Verification items for this drawing (mm, ordinates from the low corner). A direction names the side the tool comes from. Round coordinates to 2 decimals unless told otherwise and drop trailing zeros. Order: outer loops, then holes, each group sorted by start corner. A loop starts at its lowest first (then second) coordinate and runs counter-clockwise, first axis right, second up. Notation, with made-up numbers: (-2.5, -6.75) -> (24.5, -6.75) arc R16 cw to (24.5, 8.25) -> close; hole circle Ø3 at (-7, 41). An arc over 180 degrees is marked (long way). Return JSON: item names as keys, results as strings. Group by question number.
Item 1: Sectioned sample at A-A on z = 268.5. Record the cut outline in (x, y).
Item 2: Sectioned sample at D-D on z = 176.5. Record the cut outline in (x, y), plus the area to 3 significant figures.
Item 3: Depth check by flat-ended pin: pin 1 Ø1 at (y, z) = (60, 263) entering from -X; pin 2 Ø6 at (x, y) = (427, 50) entering from +Z; pin 3 Ø12 at (x, y) = (158.5, 15.5) entering from -Z. Enter the tip coordinate at first touch or a pass-through.
Item 4: Draft check along Z on the marked faces 1, 2 and 3. Enter one of: pulls with the +Z half, pulls with the -Z half, needs draft (parallel to the pull), parting line crosses it, or undercut.
Item 5: Scan lines: probe 1 along X at (y, z) = (39, 124.5); probe 2 along X at (y, z) = (17, 221.5); probe 3 along X at (y, z) = (36, 222). Record each from-to range of solid material in increasing order. Write a range as from..to.
Item 6: Access from +Z, -Z, +X, -X, +Y, -Y to the whole of each face (thin tool, end or side, straight path). Record for the marked faces 4, 5, 6, 7 and 8.
Item 7: Sectioned sample at C-C on y = 86.5. Record the cut outline in (x, z), plus the area to 3 significant figures.
Item 8: Sectioned sample at B-B on x = 91.5. Record the cut outline in (y, z).
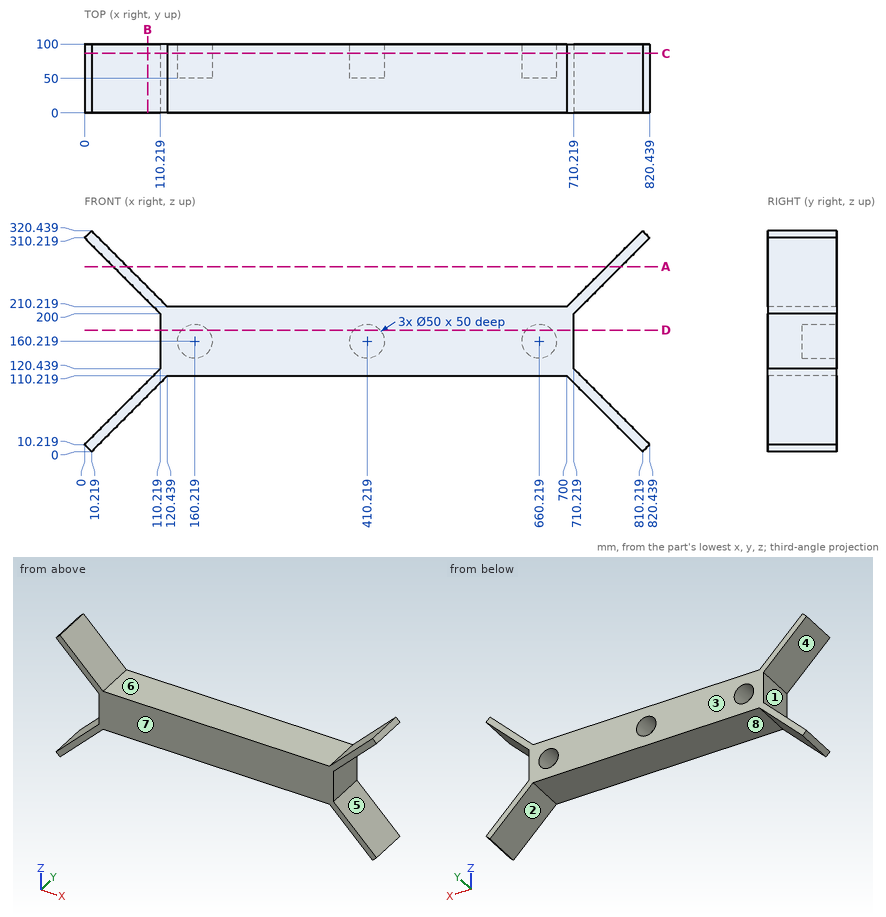
Recorded:
{
 "1": {"outline": "(41.72, 0) -> (62.16, 0) -> (62.16, 100) -> (41.72, 100) -> close; (758.28, 0) -> (778.72, 0) -> (778.72, 100) -> (758.28, 100) -> close"},
 "2": {"outline": "(110.22, 0) -> (710.22, 0) -> (710.22, 100) -> (679.19, 100) -> (679.19, 50) -> (641.25, 50) -> (641.25, 100) -> (429.19, 100) -> (429.19, 50) -> (391.25, 50) -> (391.25, 100) -> (179.19, 100) -> (179.19, 50) -> (141.25, 50) -> (141.25, 100) -> (110.22, 100) -> close", "area": "54,300 mm²"},
 "3": {"pin 1": "x = 46.72", "pin 2": "z = 210.22", "pin 3": "z = 110.22"},
 "4": {"face 1": "undercut", "face 2": "pulls with the -Z half", "face 3": "needs draft"},
 "5": {"probe 1": "110.22..710.22", "probe 2": "88.72..109.16, 711.28..731.72", "probe 3": "88.22..108.66, 711.78..732.22"},
 "6": {"face 4": "-X, +Y, -Y", "face 5": "+X, +Y, -Y", "face 6": "+Z, +Y, -Y", "face 7": "+Z, -Z, +X, -X, -Y", "face 8": "-Z, +Y, -Y"},
 "7": {"outline": "(0, 10.22) -> (10.22, 0) -> (120.44, 110.22) -> (700, 110.22) -> (810.22, 0) -> (820.44, 10.22) -> (710.22, 120.44) -> (710.22, 200) -> (820.44, 310.22) -> (810.22, 320.44) -> (700, 210.22) -> (120.44, 210.22) -> (10.22, 320.44) -> (0, 310.22) -> (110.22, 200) -> (110.22, 120.44) -> close; hole circle Ø50 at (160.22, 160.22); hole circle Ø50 at (410.22, 160.22); hole circle Ø50 at (660.22, 160.22)", "area": "62,900 mm²"},
 "8": {"outline": "(0, 81.28) -> (100, 81.28) -> (100, 101.72) -> (0, 101.72) -> close; (0, 218.72) -> (100, 218.72) -> (100, 239.16) -> (0, 239.16) -> close"}
}
